Build history of the part. All positions in model axes, mm. A direction names the side the tool comes from. Give positions to 0.01 mm unless a question says otherwise; leave off trailing zeros. Loops run counter-clockwise (first coordinate to the right, second up) from the corner with the lowest first, then second, coordinate; pieces in that order, holes last. Notation, with made-up numbers: (68.25, 74) -> (103.25, 74) arc R5 ccw to (103.25, 80) -> close; hole circle Ø8 at (15.25, 61). An arc over 180 degrees is marked (long way). Answer in a Markdown table with one row per item. Add a question column.
from build123d import *

# Parameters (mm, degrees)
BOSS_EXTRUDE1_DEPTH = 100
SKETCH2_R           = 3
CUT_EXTRUDE1_DEPTH  = 4.5
SKETCH3_R           = 1.75
CUT_EXTRUDE2_DEPTH  = 4.5
LPATTERN1_COUNT     = 4
LPATTERN1_PITCH     = 25


with BuildPart() as part:
    # Sketch1 → Boss-Extrude1 (new body)
    with BuildSketch(Plane.XY):
        with BuildLine():
            Line((6, -3.5), (6, 0.368911094))
            ThreePointArc((6, 0.368911094), (5.63354293, 0.61854293), (5.383911094, 0.985))
            Line((5.383911094, 0.985), (4.92112495, 0.985))
            ThreePointArc((4.92112495, 0.985), (4.265, 1.46), (4.92112495, 1.935))
            Line((4.92112495, 1.935), (5.383911094, 1.935))
            ThreePointArc((5.383911094, 1.935), (5.63354293, 2.30145707), (6, 2.551088906))
            Line((6, 2.551088906), (6, 3.5))
            Line((6, 3.5), (5.5, 4))
            Line((5.5, 4), (-5.5, 4))
            Line((-5.5, 4), (-6, 3.5))
            Line((-6, 3.5), (-6, 2.551088906))
            ThreePointArc((-6, 2.551088906), (-5.63354293, 2.30145707), (-5.383911094, 1.935))
            Line((-5.383911094, 1.935), (-4.92112495, 1.935))
            ThreePointArc((-4.92112495, 1.935), (-4.265, 1.46), (-4.92112495, 0.985))
            Line((-4.92112495, 0.985), (-5.383911094, 0.985))
            ThreePointArc((-5.383911094, 0.985), (-5.63354293, 0.61854293), (-6, 0.368911094))
            Line((-6, 0.368911094), (-6, -3.5))
            Line((-6, -3.5), (-5.5, -4))
            Line((-5.5, -4), (5.5, -4))
            Line((5.5, -4), (6, -3.5))
        make_face()
    extrude(amount=BOSS_EXTRUDE1_DEPTH)

    # Sketch2 → Cut-Extrude1 (cut)
    with BuildSketch(Plane(origin=(0, 4, 0), x_dir=(1, 0, 0), z_dir=(0, 1, 0))):
        with Locations((0, -12.5)):
            Circle(SKETCH2_R)
    cut_extrude1 = extrude(amount=-CUT_EXTRUDE1_DEPTH, mode=Mode.SUBTRACT)

    # Sketch3 → Cut-Extrude2 (cut, through all)
    with BuildSketch(Plane(origin=(0, -0.5, 0), x_dir=(1, 0, 0), z_dir=(0, 1, 0))):
        with Locations((0, -12.5)):
            Circle(SKETCH3_R)
    cut_extrude2 = extrude(amount=-CUT_EXTRUDE2_DEPTH, mode=Mode.SUBTRACT)

    # LPattern1: Cut-Extrude1, Cut-Extrude2 ×4
    with Locations(*[(0, 0, i * LPATTERN1_PITCH) for i in range(1, LPATTERN1_COUNT)]):
        add(cut_extrude1, mode=Mode.SUBTRACT)
        add(cut_extrude2, mode=Mode.SUBTRACT)


solid = part.part
(1) Flat gauge pin, fed straight in: pin 1 Ø4 at (x, z) = (0, 37.5) entering from +Y. Where does the tip first touch, or does it go through?
(2) Saw through at A-A, the plane z = 62.5. List the corners of the cut face in (x, y) (3 decimals).
(3) Saw through at B-B, the plane x = 0. State how many separate pieces and enclosed holes the cut face has, then the cut area to 3 significant figures.
(4) Two-plate mould, pull along X, no slides. Class faces 1 (the flat face through (0, -4, 49)), 2 (the flat face through (6, -2, 49)), 3 (the flat face through (2, -0.5, 62)): released by +X, released by -X, zero draft, split by the parting line, or undercut.
(5) Wall check: line 1 along Z through (x, y) = (0, -3.05); line 2 along Z through (x, y) = (0, 3.1); line 3 along X through (y, z) = (2.95, 37.5). Give the ranges that are in metal, low to high. Write a range as from..to.
(6) 3-axis set-ups, long thin cutter, end or side, ignore diameter. For faces 4 (the flat face through (0, -0.5, 14.5)), 5 (the flat face through (-6, -2, 49)): which of +Z, -Z, +X, -X, +Y, -Y reach the whole face in a straight line?
Worked answers:
| question | item | result |
|---|---|---|
| 1 | pin 1 | y = -0.5 |
| 2 | outline | (-6, -3.5) -> (-5.5, -4) -> (-1.75, -4) -> (-1.75, -0.5) -> (-3, -0.5) -> (-3, 4) -> (-5.5, 4) -> (-6, 3.5) -> (-6, 2.551) arc R1.19 cw to (-5.384, 1.935) -> (-4.921, 1.935) arc R0.5 cw (long way) to (-4.921, 0.985) -> (-5.384, 0.985) arc R1.19 cw to (-6, 0.369) -> close; (1.75, -4) -> (5.5, -4) -> (6, -3.5) -> (6, 0.369) arc R1.19 cw to (5.384, 0.985) -> (4.921, 0.985) arc R0.5 cw (long way) to (4.921, 1.935) -> (5.384, 1.935) arc R1.19 cw to (6, 2.551) -> (6, 3.5) -> (5.5, 4) -> (3, 4) -> (3, -0.5) -> (1.75, -0.5) -> close |
| 3 | separate pieces | 5 |
| 3 | enclosed holes | 0 |
| 3 | area | 643 mm^2 |
| 4 | face 1 | zero draft |
| 4 | face 2 | released by +X |
| 4 | face 3 | undercut |
| 5 | line 1 | 0..10.75, 14.25..35.75, 39.25..60.75, 64.25..85.75, 89.25..100 |
| 5 | line 2 | 0..9.5, 15.5..34.5, 40.5..59.5, 65.5..84.5, 90.5..100 |
| 5 | line 3 | -6..-3, 3..6 |
| 6 | face 4 | +Y |
| 6 | face 5 | +Z, -Z, -X, +Y, -Y |
